Source: CAD feature listing. Evaluate the final solid. Frame: model axes, mm. Face numbers are marked on the shaded views. A direction names the side the tool comes from. Round coordinates to 2 decimals unless told otherwise and drop trailing zeros. Order: outer loops, then holes, each group sorted by start corner. A loop starts at its lowest first (then second) coordinate and runs counter-clockwise, first axis right, second up. Notation, with made-up numbers: (-10, -25) -> (45, -25) arc R11 ccw to (45, -16) -> close; hole circle Ø9 at (75.5, 1). An arc over 180 degrees is marked (long way). One line per item, written item: value. Start each with the question number.
1) Reachability of the marked faces 1, 2, 3 and 4 from +Z, -Z, +X, -X, +Y, -Y: full face, straight path, thin tool, end or side. Return the list, or none.
2) Section B-B (x = 23). Return the cut outline in (y, z), and give its area (3 significant figures).
3) Section C-C (z = -10). Return the cut outline in (x, y).
4) Pin query (flat end, axial travel): P1, Ø4, axis at x = 122, z = 130, coming from the +Y side; P2, Ø10, axis at y = 9, z = 14.5, coming from the +X side; P3, Ø9, axis at y = 8, z = 124, coming from the +X side; P4, Ø0.9, axis at x = 68.5, z = 60.5, coming from the +Y side. Return the tip coordinate at first contact, or that it passes through.
5) Ray query, L1, parallel to X at y = 3, z = 65; L2, parallel to Z at x = 122, y = 0.75; L3, parallel to Z at x = 122, y = 2. Return the intervals inside material, ascending.
6) Mould query, pull axis X, two halves, no side actions, for the marked faces 5 and 6. Classes: pulls with the +X half, pulls with the -X half, needs draft (parallel to the pull), parting line crosses it, or undercut.
7) Section A-A (y = 8.5). State how many separate pieces and enclosed holes the cut face has, and give its area (3 significant figures).
```python
from build123d import *

# Parameters (mm, degrees)
SKETCH1_W              = 130.485281374
SKETCH1_H              = 138.485281374
SKETCH1_R              = 1.5
BOSS_EXTRUDE1_DEPTH    = 1.5
CUT_EXTRUDE1_DEPTH     = 17.5
BOSS_EXTRUDE2_DEPTH    = 138.485281
SKETCH14_R             = 3
SKETCH14_R_2           = 1.5
BOSS_EXTRUDE7_DEPTH    = 3
SKETCH15_R             = 1.5
CUT_EXTRUDE6_DEPTH     = 3
SKETCH16_R             = 3
SKETCH16_R_2           = 1.5
BOSS_EXTRUDE8_DEPTH    = 3
SKETCH17_R             = 1.5
CUT_EXTRUDE7_DEPTH     = 3
SKETCH18_R             = 3.5
SKETCH18_R_2           = 1.5
BOSS_EXTRUDE9_DEPTH    = 24.5
SKETCH19_W             = 20
SKETCH19_H             = 2
BOSS_EXTRUDE10_DEPTH   = 28
BOSS_EXTRUDE11_DEPTH   = 20
SKETCH24_R             = 1.5
CUT_EXTRUDE9_DEPTH     = 16
BOSS_EXTRUDE13_DEPTH   = 40
SKETCH27_W             = 17
SKETCH27_H             = 2
BOSS_EXTRUDE13_2_DEPTH = 40
SKETCH28_W             = 29.536458096
SKETCH28_H             = 15.843310856
CUT_EXTRUDE10_DEPTH    = 20
BOSS_EXTRUDE14_DEPTH   = 18
CUT_EXTRUDE11_DEPTH    = 26
BOSS_EXTRUDE15_DEPTH   = 2
FILLET1_R              = 10
SKETCH33_W             = 20
SKETCH33_H             = 2
BOSS_EXTRUDE16_DEPTH   = 28
BOSS_EXTRUDE17_DEPTH   = 20
CUT_EXTRUDE12_DEPTH    = 20


with BuildPart() as part:
    # Sketch1 → Boss-Extrude1 (new body)
    with BuildSketch(Plane(origin=(0, 0, 0), x_dir=(1, 0, 0), z_dir=(0, 1, 0))):
        with Locations((61, -65)):
            Rectangle(SKETCH1_W, SKETCH1_H)
        Circle(SKETCH1_R, mode=Mode.SUBTRACT)
        with Locations((122, 0)):
            Circle(SKETCH1_R, mode=Mode.SUBTRACT)
        with Locations((0, -130)):
            Circle(SKETCH1_R, mode=Mode.SUBTRACT)
        with Locations((122, -130)):
            Circle(SKETCH1_R, mode=Mode.SUBTRACT)
    extrude(amount=BOSS_EXTRUDE1_DEPTH)

    # Sketch3 → Cut-Extrude1 (cut)
    with BuildSketch(Plane(origin=(0, 1.5, 0), x_dir=(1, 0, 0), z_dir=(0, 1, 0))):
        Polygon((15.757359313, -65), (15.757359313, 4.242640687), (106.242640687, 4.242640687), (106.242640687, -65), (106.242640687, -134.242640687), (15.757359313, -134.242640687), align=None)
    extrude(amount=-CUT_EXTRUDE1_DEPTH, mode=Mode.SUBTRACT)

    # Sketch4 → Boss-Extrude2 (add, through all)
    with BuildSketch(Plane.XY.offset(134.242640687)):
        Polygon((15.757359313, 0), (18.757359313, -6), (103.242640687, -6), (106.242640687, 0), (106.242640687, 1.5), (104.742640687, 1.5), (101.703883411, -4.5), (83.627274603, -4.5), (38.372725397, -4.5), (20.296116589, -4.5), (17.257359313, 1.5), (15.757359313, 1.5), align=None)
    extrude(amount=-BOSS_EXTRUDE2_DEPTH)

    # Sketch14 → Boss-Extrude7 (add)
    with BuildSketch(Plane(origin=(0, 1.5, 0), x_dir=(1, 0, 0), z_dir=(0, 1, 0))):
        with Locations((0, -130)):
            Circle(SKETCH14_R)
        with Locations((0, -130)):
            Circle(SKETCH14_R_2, mode=Mode.SUBTRACT)
        with Locations((122, -130)):
            Circle(SKETCH14_R)
        with Locations((122, -130)):
            Circle(SKETCH14_R_2, mode=Mode.SUBTRACT)
    extrude(amount=BOSS_EXTRUDE7_DEPTH)

    # Sketch15 → Cut-Extrude6 (cut)
    with BuildSketch(Plane(origin=(0, 1.5, 0), x_dir=(1, 0, 0), z_dir=(0, 1, 0))):
        with Locations((0, -65)):
            Circle(SKETCH15_R)
        with Locations((122, -65)):
            Circle(SKETCH15_R)
    extrude(amount=-CUT_EXTRUDE6_DEPTH, mode=Mode.SUBTRACT)

    # Sketch16 → Boss-Extrude8 (add)
    with BuildSketch(Plane(origin=(0, 1.5, 0), x_dir=(1, 0, 0), z_dir=(0, 1, 0))):
        with Locations((0, -65)):
            Circle(SKETCH16_R)
        with Locations((0, -65)):
            Circle(SKETCH16_R_2, mode=Mode.SUBTRACT)
        with Locations((122, -65)):
            Circle(SKETCH16_R)
        with Locations((122, -65)):
            Circle(SKETCH16_R_2, mode=Mode.SUBTRACT)
    extrude(amount=BOSS_EXTRUDE8_DEPTH)

    # Sketch17 → Cut-Extrude7 (cut)
    with BuildSketch(Plane(origin=(0, 1.5, 0), x_dir=(1, 0, 0), z_dir=(0, 1, 0))):
        with Locations((0, -50)):
            Circle(SKETCH17_R)
        with Locations((0, -80)):
            Circle(SKETCH17_R)
        with Locations((122, -80)):
            Circle(SKETCH17_R)
        with Locations((122, -50)):
            Circle(SKETCH17_R)
    extrude(amount=-CUT_EXTRUDE7_DEPTH, mode=Mode.SUBTRACT)

    # Sketch18 → Boss-Extrude9 (add)
    with BuildSketch(Plane(origin=(0, -4.5, 0), x_dir=(1, 0, 0), z_dir=(0, 1, 0))):
        with Locations((53.22, -60)):
            Circle(SKETCH18_R)
        with Locations((53.22, -60)):
            Circle(SKETCH18_R_2, mode=Mode.SUBTRACT)
        with Locations((68.78, -60)):
            Circle(SKETCH18_R)
        with Locations((68.78, -60)):
            Circle(SKETCH18_R_2, mode=Mode.SUBTRACT)
    extrude(amount=BOSS_EXTRUDE9_DEPTH)

    # Sketch19 → Boss-Extrude10 (add)
    with BuildSketch(Plane(origin=(0, -4.5, 0), x_dir=(1, 0, 0), z_dir=(0, 1, 0))):
        with Locations((61, -110.242640687)):
            Rectangle(SKETCH19_W, SKETCH19_H)
        with Locations((61, -103.242640687)):
            Rectangle(SKETCH19_W, SKETCH19_H)
    extrude(amount=BOSS_EXTRUDE10_DEPTH)

    # Sketch20 → Boss-Extrude11 (add)
    with BuildSketch(Plane(origin=(71, 0, 0), x_dir=(0, 0, -1), z_dir=(1, 0, 0))):
        Polygon((-111.242640687, -4.5), (-118.242640687, -4.5), (-111.242640687, 15.5), align=None)
        Polygon((-115.329396397, -2.668636481), (-111.803828851, -2.668636481), (-111.803828851, 10.297263435), (-116.337361542, -2.040762337), align=None, mode=Mode.SUBTRACT)
        Polygon((-95.242640687, -4.5), (-102.242640687, 15.5), (-102.242640687, -4.5), align=None)
        Polygon((-101.681452524, 10.297263435), (-97.147919832, -2.040762337), (-98.155884977, -2.668636481), (-101.681452524, -2.668636481), align=None, mode=Mode.SUBTRACT)
    extrude(amount=-BOSS_EXTRUDE11_DEPTH)

    # Sketch24 → Cut-Extrude9 (cut)
    with BuildSketch(Plane(origin=(0, -4.5, 0), x_dir=(1, 0, 0), z_dir=(0, 1, 0))):
        with Locations((61, -65)):
            Circle(SKETCH24_R)
    extrude(amount=-CUT_EXTRUDE9_DEPTH, mode=Mode.SUBTRACT)



with BuildPart() as body_2:
    # Sketch27 → Boss-Extrude13 (new body)
    with BuildSketch(Plane(origin=(0, -4.5, 0), x_dir=(1, 0, 0), z_dir=(0, 1, 0))):
        Polygon((52.5, 14.242640687), (61, 14.242640687), (69.5, 14.242640687), (69.5, 16.242640687), (52.5, 16.242640687), align=None)
    extrude(amount=BOSS_EXTRUDE13_DEPTH)


with BuildPart() as body_3:
    # Sketch27 → Boss-Extrude13 2 (new body)
    with BuildSketch(Plane(origin=(0, -4.5, 0), x_dir=(1, 0, 0), z_dir=(0, 1, 0))):
        with Locations((61, 23.742640687)):
            Rectangle(SKETCH27_W, SKETCH27_H)
    extrude(amount=BOSS_EXTRUDE13_2_DEPTH)


with BuildPart() as cut_extrude10_tool:
    # Sketch28 → Cut-Extrude10 (new body)
    with BuildSketch(Plane.XZ.offset(4.5)):
        with Locations((60.962328077, -18.662784731)):
            Rectangle(SKETCH28_W, SKETCH28_H)
    extrude(amount=-CUT_EXTRUDE10_DEPTH)


with BuildPart() as body_2_1:
    add(body_2.part)

    # Cut-Extrude10: cut by cut_extrude10_tool
    add(cut_extrude10_tool.part, mode=Mode.SUBTRACT)


with BuildPart() as body_3_1:
    add(body_3.part)

    # Cut-Extrude10: cut by cut_extrude10_tool
    add(cut_extrude10_tool.part, mode=Mode.SUBTRACT)


with BuildPart() as part_1:
    add(part.part)

    add(body_2_1.part)  # Boss-Extrude14 merges body 2

    add(body_3_1.part)  # Boss-Extrude14 merges body 3
    # Sketch29 → Boss-Extrude14 (add)
    with BuildSketch(Plane.ZY.offset(-52.5)):
        Polygon((-24.742640687, 13.5), (-4.242640687, -6), (4.73835691, -5.480059004), (-14.241702094, 13.5), (-14.241702094, 15.5), (-24.742640687, 15.5), align=None)
    extrude(amount=-BOSS_EXTRUDE14_DEPTH)

    # Sketch30 → Cut-Extrude11 (cut)
    with BuildSketch(Plane.ZY.offset(-51)):
        Polygon((111.242640687, 15.5), (111.242640687, -4.5), (118.242640687, -4.5), align=None)
    extrude(amount=-CUT_EXTRUDE11_DEPTH, mode=Mode.SUBTRACT)

    # Sketch32 → Boss-Extrude15 (add)
    with BuildSketch(Plane.XY.offset(111.242640687)):
        Polygon((71, 23.5), (77.545089148, -4.5), (71, -4.5), align=None)
        Polygon((51, -4.5), (51, 23.5), (44.454910852, -4.5), align=None)
    extrude(amount=-BOSS_EXTRUDE15_DEPTH)

    # Fillet1
    fillet1_edges = [part_1.edges().sort_by_distance(p)[0] for p in [
        (77.545089148, -4.5, 110.242640687),
        (44.454910852, -4.5, 110.242640687),
    ]]
    fillet(fillet1_edges, radius=FILLET1_R)

    # Sketch33 → Boss-Extrude16 (add)
    with BuildSketch(Plane(origin=(0, -4.5, 0), x_dir=(1, 0, 0), z_dir=(0, 1, 0))):
        with Locations((61, -117.27180301)):
            Rectangle(SKETCH33_W, SKETCH33_H)
    extrude(amount=BOSS_EXTRUDE16_DEPTH)

    # Sketch34 → Boss-Extrude17 (add)
    with BuildSketch(Plane(origin=(71, 0, 0), x_dir=(0, 0, -1), z_dir=(1, 0, 0))):
        Polygon((-118.27180301, -4.5), (-118.27180301, 15.5), (-127.27180301, -4.5), align=None)
    extrude(amount=-BOSS_EXTRUDE17_DEPTH)

    # Sketch35 → Cut-Extrude12 (cut)
    with BuildSketch(Plane(origin=(71, 0, 0), x_dir=(0, 0, -1), z_dir=(1, 0, 0))):
        Polygon((-121.77180301, -2.5), (-118.236471352, -2.5), (-118.236471352, 10.68955001), (-123.840420038, -2.5), align=None)
    extrude(amount=-CUT_EXTRUDE12_DEPTH, mode=Mode.SUBTRACT)


solid = part_1.part
```
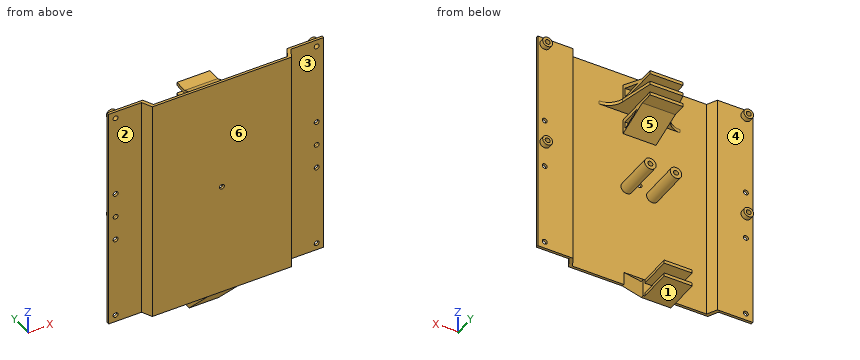
Findings:
1. face 1: -Z, +X, -X, +Y, -Y
1. face 2: +Z, -Z, -X, -Y
1. face 3: +Z, -Z, +X, -Y
1. face 4: +Y
2. outline: (-6, -4.24) -> (-4.5, -4.24) -> (-4.5, 134.24) -> (-6, 134.24) -> close
2. area: 208 mm2
3. outline: (52.5, -0.52) -> (70.5, -0.52) -> (70.5, 9.26) -> (52.5, 9.26) -> close
4. P1: y = 4.5
4. P2: through
4. P3: x = 71
4. P4: y = -4.5
5. L1: -3 to -1.5, 1.5 to 3, 119 to 120.5, 123.5 to 125
5. L2: -4.24 to -1.5, 1.5 to 48.5, 51.5 to 63.5, 66.5 to 78.5, 81.5 to 128.5, 131.5 to 134.24
5. L3: 62 to 63.5, 66.5 to 68, 127 to 128.5, 131.5 to 133
6. face 5: undercut
6. face 6: needs draft
7. separate pieces: 8
7. enclosed holes: 2
7. area: 461 mm2
